Autodesk Inventor part; units mm, degrees
ref_plane "YZ Plane" through (0, 0, 0) normal (1, 0, 0) x (0, 1, 0)
ref_plane "XZ Plane" through (0, 0, 0) normal (0, 1, 0) x (-1, 0, 0)
ref_plane "XY Plane" through (0, 0, 0) normal (0, 0, 1) x (1, 0, 0)
sketch "Sketch1" plane through (0, 0, 0) normal (0, 0, 1) x (1, 0, 0)
  line L0 (0.75, -26.5) -> (0.75, 26.5)
  line L1 (0.75, 26.5) -> (-0.75, 26.5)
  line L2 (-0.75, 26.5) -> (-0.75, -26.5)
  line L3 (-0.75, -26.5) -> (0.75, -26.5)
  line L4 (27.75, 26.5) -> (27.75, -26.5)
  line L5 (27.75, -26.5) -> (29.25, -26.5)
  line L6 (29.25, -26.5) -> (29.25, 26.5)
  line L7 (29.25, 26.5) -> (27.75, 26.5)
  line L8 (35.75, -26.5) -> (35.75, 26.5)
  line L9 (35.75, 26.5) -> (34.25, 26.5)
  line L10 (34.25, 26.5) -> (34.25, -26.5)
  line L11 (34.25, -26.5) -> (35.75, -26.5)
  line L12 (64.25, -26.5) -> (64.25, 26.5)
  line L13 (62.75, 26.5) -> (62.75, -26.5)
  line L14 (62.75, -26.5) -> (64.25, -26.5)
  line L15 (64.25, -26.5) -> (64.25, 26.5)
  line L16 (64.25, 26.5) -> (62.75, 26.5)
  line L17 (64.25, -26.5) -> (-0.75, -26.5)
  line L18 (-0.75, -26.5) -> (-0.75, 18.5)
  line L19 (-0.75, 18.5) -> (64.25, 18.5)
  line L20 (64.25, 18.5) -> (64.25, -26.5)
  line L21 (62.75, 18.5) -> (62.75, -26.5)
  line L22 (35.75, 18.5) -> (35.75, -26.5)
  line L23 (34.25, 18.5) -> (34.25, -26.5)
  line L24 (29.25, 18.5) -> (29.25, -26.5)
  line L25 (27.75, -26.5) -> (27.75, 18.5)
  line L26 (0.75, 18.5) -> (0.75, -26.5)
  point P0 (0, 0)
  dimension "d0" = 45
extrude "Extrusion1" add sketch "Sketch1" along normal blind 3 contours L3 L2 L19 L0 | L0 L19 L4 L17 | L4 L19 L6 L5 | L6 L19 L10 L17 | L10 L19 L8 L11 | L8 L19 L13 L17 | L13 L19 L12 L14
sketch "Sketch2" plane through (0, 0, 3) normal (0, 0, 1) x (1, 0, 0)
  line L0 (0.75, -26.5) -> (0.75, 26.5)
  line L1 (0.75, 26.5) -> (-0.75, 26.5)
  line L2 (-0.75, 26.5) -> (-0.75, -26.5)
  line L3 (-0.75, -26.5) -> (0.75, -26.5)
  line L4 (27.75, 26.5) -> (27.75, -26.5)
  line L5 (27.75, -26.5) -> (29.25, -26.5)
  line L6 (29.25, -26.5) -> (29.25, 26.5)
  line L7 (29.25, 26.5) -> (27.75, 26.5)
  line L8 (35.75, -26.5) -> (35.75, 26.5)
  line L9 (35.75, 26.5) -> (34.25, 26.5)
  line L10 (34.25, 26.5) -> (34.25, -26.5)
  line L11 (34.25, -26.5) -> (35.75, -26.5)
  line L12 (64.25, -26.5) -> (64.25, 26.5)
  line L13 (62.75, 26.5) -> (62.75, -26.5)
  line L14 (62.75, -26.5) -> (64.25, -26.5)
  line L15 (64.25, -26.5) -> (64.25, 26.5)
  line L16 (64.25, 26.5) -> (62.75, 26.5)
  line L17 (64.25, -26.5) -> (-0.75, -26.5)
  line L18 (-0.75, -26.5) -> (-0.75, 18.5)
  line L19 (-0.75, 18.5) -> (64.25, 18.5)
  line L20 (64.25, 18.5) -> (64.25, -26.5)
  line L21 (62.75, 18.5) -> (62.75, -26.5)
  line L22 (35.75, 18.5) -> (35.75, -26.5)
  line L23 (34.25, 18.5) -> (34.25, -26.5)
  line L24 (29.25, 18.5) -> (29.25, -26.5)
  line L25 (27.75, -26.5) -> (27.75, 18.5)
  line L26 (0.75, 18.5) -> (0.75, -26.5)
  line L27 (0.75, -26.5) -> (0.75, 26.5)
  line L28 (0.75, 26.5) -> (-0.75, 26.5)
  line L29 (-0.75, 26.5) -> (-0.75, -26.5)
  line L30 (-0.75, -26.5) -> (0.75, -26.5)
  line L31 (27.75, 26.5) -> (27.75, -26.5)
  line L32 (27.75, -26.5) -> (29.25, -26.5)
  line L33 (29.25, -26.5) -> (29.25, 26.5)
  line L34 (29.25, 26.5) -> (27.75, 26.5)
  line L35 (35.75, -26.5) -> (35.75, 26.5)
  line L36 (35.75, 26.5) -> (34.25, 26.5)
  line L37 (34.25, 26.5) -> (34.25, -26.5)
  line L38 (34.25, -26.5) -> (35.75, -26.5)
  line L39 (64.25, -26.5) -> (64.25, 26.5)
  line L40 (62.75, 26.5) -> (62.75, -26.5)
  line L41 (62.75, -26.5) -> (64.25, -26.5)
  line L42 (64.25, -26.5) -> (64.25, 26.5)
  line L43 (64.25, 26.5) -> (62.75, 26.5)
  line L44 (64.25, -26.5) -> (-0.75, -26.5)
  line L45 (-0.75, -26.5) -> (-0.75, 18.5)
  line L46 (-0.75, 18.5) -> (64.25, 18.5)
  line L47 (64.25, 18.5) -> (64.25, -26.5)
  line L48 (62.75, 18.5) -> (62.75, -26.5)
  line L49 (35.75, 18.5) -> (35.75, -26.5)
  line L50 (34.25, 18.5) -> (34.25, -26.5)
  line L51 (29.25, 18.5) -> (29.25, -26.5)
  line L52 (27.75, -26.5) -> (27.75, 18.5)
  line L53 (0.75, 18.5) -> (0.75, -26.5)
  point P0 (0, 0)
  point P1 (0, 0)
  point P2 (0, 0)
  dimension "d3" = 45
  dimension "d4" = 45
extrude "Extrusion2" add sketch "Sketch2" along normal blind 3 contours L3 L2 L19 L0 | L4 L19 L6 L5 | L10 L19 L8 L11 | L13 L19 L12 L14
properties part number "base_2"
Geometry: final body of the model. Coordinates: model frame, mm. A direction names the side the tool comes from. Round coordinates to 2 decimals unless told otherwise and drop trailing zeros. Order: outer loops, then holes, each group sorted by start corner. A loop starts at its lowest first (then second) coordinate and runs counter-clockwise, first axis right, second up. Notation, with made-up numbers: (-37.5, 81.25) -> (-28.5, 81.25) arc R28 cw to (-28.5, 113.25) -> close; hole circle Ø2 at (17.25, -15.75). An arc over 180 degrees is marked (long way). Use one line per item in the form item = value.
(1) Ray query, probe 1 along X at (y, z) = (-13, 3.8); probe 2 along Z at (x, y) = (7.5, -4). Return the intervals inside material, ascending. Write a range as [from, to].
Results list:
probe_1 = [-0.75, 0.75], [27.75, 29.25], [34.25, 35.75], [62.75, 64.25]
probe_2 = [0, 3]
(2) Draft query along X for faces 3 (the face through (27.75, -4, 4)), 4 (the face through (64.25, -4, 3)), 5 (the face through (35, -4, 6)). Return one class per face: pulls with the +X half, pulls with the -X half, needs draft (parallel to the pull), parting line crosses it, or undercut.
Results list:
face_3 = undercut
face_4 = pulls with the +X half
face_5 = needs draft
(3) Access query for faces 1 (the face through (-0.75, -4, 3)), 2 (the face through (34.25, -4, 4)). Directions: +Z, -Z, +X, -X, +Y, -Y. A direction counts if a zero-diameter tool reaches every point of the face in a straight line with its end or side. Return the directions, or none.
Results list:
face_1 = +Z, -Z, -X, +Y, -Y
face_2 = +Z, +Y, -Y
(4) Section B-B on y = 5. Return loops of the section in (x, z).
Results list:
outline = (-0.75, 0) -> (64.25, 0) -> (64.25, 6) -> (62.75, 6) -> (62.75, 3) -> (35.75, 3) -> (35.75, 6) -> (34.25, 6) -> (34.25, 3) -> (29.25, 3) -> (29.25, 6) -> (27.75, 6) -> (27.75, 3) -> (0.75, 3) -> (0.75, 6) -> (-0.75, 6) -> close
(5) Section C-C on x = 27. Return loops of the section in (y, z).
Results list:
outline = (-26.5, 0) -> (18.5, 0) -> (18.5, 3) -> (-26.5, 3) -> close
(6) Section A-A on z = 4.1. Return loops of the section in (x, y), and give its area (3 significant figures).
Results list:
outline = (-0.75, -26.5) -> (0.75, -26.5) -> (0.75, 18.5) -> (-0.75, 18.5) -> close; (27.75, -26.5) -> (29.25, -26.5) -> (29.25, 18.5) -> (27.75, 18.5) -> close; (34.25, -26.5) -> (35.75, -26.5) -> (35.75, 18.5) -> (34.25, 18.5) -> close; (62.75, -26.5) -> (64.25, -26.5) -> (64.25, 18.5) -> (62.75, 18.5) -> close
area = 270 mm^2
(7) First-contact query: pin 1 Ø8 at (x, y) = (29.5, -11.5) entering from +Z; pin 2 Ø13.5 at (x, y) = (46.5, -1) entering from +Z. Flat tips, straight axial feed; report the tip coordinate or a pass-through.
Results list:
pin_1 = 6
pin_2 = 3
